```python
from build123d import *

# Parameters (mm, degrees)
F1_DEPTH = 15


with BuildPart() as f1:
    # F0 (on Front) → F1 (new body)
    with BuildSketch(Plane.XZ):
        with BuildLine():
            ThreePointArc((0, 40.1), (28.354982, 28.354982), (40.1, 0))
            Line((40.1, 0), (42.808995, 0))
            ThreePointArc((42.808995, 0), (46.54398, 1.675863), (47.775236, 5.580046))
            ThreePointArc((47.775236, 5.580046), (38.187671, 29.245715), (17.838656, 44.669815))
            ThreePointArc((17.838656, 44.669815), (16.387117, 45.562084), (15.31947, 46.889954))
            Line((15.31947, 46.889954), (9.427711, 57.523294))
            ThreePointArc((9.427711, 57.523294), (7.592257, 59.407927), (5.054194, 60.1))
            Line((5.054194, 60.1), (0, 60.1))
            Line((0, 60.1), (0, 40.1))
        make_face()
    extrude(amount=F1_DEPTH)


solid = f1.part
```
The listing builds one solid part. Answer for the finished solid, in the listing's coordinates (mm). Round coordinates to 2 decimals unless told otherwise and drop trailing zeros. Loops run counter-clockwise (first coordinate to the right, second up) from the corner with the lowest first, then second, coordinate; pieces in that order, holes last. Notation, with made-up numbers: (-14, 70) -> (25, 70) arc R23 ccw to (25, 96) -> close; hole circle Ø8 at (67.5, 88). An arc over 180 degrees is marked (long way). Use one line per item in the form item = value.
1. The part is cut by section C-C on x = 24.5. Determine the outline of the cut face in (y, z), and give its area (3 significant figures).
Answer key:
outline = (-15, 31.75) -> (0, 31.75) -> (0, 41.39) -> (-15, 41.39) -> close
area = 145 mm²
2. Flat-ended cylindrical pins translate along their axes: pin 1 Ø1 at (y, z) = (-13, 33.5) entering from +X; pin 2 Ø2 at (x, y) = (29, -13) entering from +Z; pin 3 Ø2 at (y, z) = (-9, 33.5) entering from -X; pin 4 Ø1 at (x, z) = (20, 33) entering from +Y. Find the tip coordinate at first contact, or state that the pin passes through.
Answer key:
pin_1 = 34.99
pin_2 = 39.11
pin_3 = 20.44
pin_4 = through
3. The part is cut by section B-B on z = 43. Determine the outline of the cut face in (x, y).
Answer key:
outline = (0, -15) -> (21.55, -15) -> (21.55, 0) -> (0, 0) -> close
4. Find the intervals of material crossed by probe 1 along X at (y, z) = (-8.5, 3); probe 2 along Z at (x, y) = (4, -2); probe 3 along Z at (x, y) = (9.5, -2.5), in increasing order. Write a range as [from, to].
Answer key:
probe_1 = [39.99, 47.39]
probe_2 = [39.9, 60.1]
probe_3 = [38.96, 57.39]
5. The part is cut by section A-A on y = -11.5. Determine the outline of the cut face in (x, z), and give its area (3 significant figures).
Answer key:
outline = (0, 40.1) arc R40.1 cw to (40.1, 0) -> (42.81, 0) arc R5 ccw to (47.78, 5.58) arc R48.1 ccw to (17.84, 44.67) arc R5 cw to (15.32, 46.89) -> (9.43, 57.52) arc R5 ccw to (5.05, 60.1) -> (0, 60.1) -> close
area = 695 mm²
